The model under review builds one solid part; all positions refer to its coordinate system, in mm. Round coordinates to 2 decimals unless told otherwise and drop trailing zeros. Loops run counter-clockwise (first coordinate to the right, second up) from the corner with the lowest first, then second, coordinate; pieces in that order, holes last. Notation, with made-up numbers: (-28.75, -28.75) -> (-3.75, -28.75) arc R35 ccw to (-3.75, 4.25) -> close; hole circle Ø11 at (8, 79). An arc over 180 degrees is marked (long way). Write each question's results on one line, items separated by ' | '. Start each with the question number.
Item 1: Clearance check with a flat-ended pin moving along its axis: pin 1 Ø2.5 at (x, z) = (-3.5, -30.75) entering from -Y. State where the tip first meets the part, or that it passes through.
Item 2: For L1, parallel to X at y = 1.8, z = -55; L2, parallel to X at y = 1.3, z = -39.5; L3, parallel to Z at x = -3.25, y = 1.35, list the stretches that pass through material, from the lowest coordinate up. Write a range as from..to.
Item 3: We need section B-B (y = 1.95). Give the number of separate pieces and of enclosed holes in the cut face, and give its area (3 significant figures).
Item 4: We need section C-C (z = 27). Give the boundary of the cut face in (x, y) (3 decimals).
Item 5: We need section A-A (z = 39.5). Give the boundary of the cut face in (x, y) (3 decimals), and give its area (3 significant figures).
from build123d import *

# Parameters (mm, degrees)
BOSS_EXTRUDE1_DEPTH = 3.175
SKETCH2_W           = 3.175
SKETCH2_H           = 15
CUT_EXTRUDE1_DEPTH  = 62.928027782
SKETCH5_R           = 1.5
CUT_EXTRUDE2_DEPTH  = 10
FILLET1_R           = 2
FILLET2_R           = 3


with BuildPart() as part:
    # Sketch1 → Boss-Extrude1 (new body)
    with BuildSketch(Plane(origin=(0, 0, 0), x_dir=(1, 0, 0), z_dir=(0, 1, 0))):
        Polygon((-15, 60), (15, 60), (15, 45), (7, 45), (7, -45), (15, -45), (15, -60), (-15, -60), (-15, -45), (-7, -45), (-7, 45), (-15, 45), align=None)
    extrude(amount=BOSS_EXTRUDE1_DEPTH)

    # Sketch2 → Cut-Extrude1 (cut, through all)
    with BuildSketch(Plane(origin=(0, 3.175, 0), x_dir=(1, 0, 0), z_dir=(0, 1, 0))):
        with Locations((7.5, 60)):
            Rectangle(SKETCH2_W, SKETCH2_H)
        with Locations((-7.5, 60)):
            Rectangle(SKETCH2_W, SKETCH2_H)
        with Locations((7.5, -60)):
            Rectangle(SKETCH2_W, SKETCH2_H)
        with Locations((-7.5, -60)):
            Rectangle(SKETCH2_W, SKETCH2_H)
    extrude(amount=-CUT_EXTRUDE1_DEPTH, mode=Mode.SUBTRACT)

    # Sketch5 → Cut-Extrude2 (cut)
    with BuildSketch(Plane.XZ):
        with Locations(Location((3.5, -39.5, 0), (0, 0, 270))):
            Circle(SKETCH5_R)
        with Locations(Location((-3.5, -39.5, 0), (0, 0, 270))):
            Circle(SKETCH5_R)
        with Locations(Location((-3.5, -30.75, 0), (0, 0, 270))):
            Circle(SKETCH5_R)
        with Locations(Location((3.5, 30.75, 0), (0, 0, 270))):
            Circle(SKETCH5_R)
        with Locations(Location((-3.5, 30.75, 0), (0, 0, 270))):
            Circle(SKETCH5_R)
        with Locations(Location((3.5, 39.5, 0), (0, 0, 270))):
            Circle(SKETCH5_R)
        with Locations(Location((-3.5, 39.5, 0), (0, 0, 270))):
            Circle(SKETCH5_R)
        with Locations(Location((3.5, -30.75, 0), (0, 0, 270))):
            Circle(SKETCH5_R)
    extrude(amount=-CUT_EXTRUDE2_DEPTH, mode=Mode.SUBTRACT)

    # Fillet1
    fillet1_edges = [part.edges().sort_by_distance(p)[0] for p in [
        (-5.9125, 1.5875, -60),
        (-9.0875, 1.5875, -60),
        (5.9125, 1.5875, 60),
        (9.0875, 1.5875, 60),
        (-5.9125, 1.5875, 60),
        (-9.0875, 1.5875, 60),
        (9.0875, 1.5875, -60),
        (5.9125, 1.5875, -60),
    ]]
    fillet(fillet1_edges, radius=FILLET1_R)

    # Fillet2
    fillet2_edges = [part.edges().sort_by_distance(p)[0] for p in [
        (7, 1.5875, -45),
        (7, 1.5875, 45),
        (15, 1.5875, 45),
        (15, 1.5875, 60),
        (-15, 1.5875, 60),
        (-15, 1.5875, 45),
        (-7, 1.5875, 45),
        (-7, 1.5875, -45),
        (-15, 1.5875, -45),
        (-15, 1.5875, -60),
        (15, 1.5875, -60),
        (15, 1.5875, -45),
    ]]
    fillet(fillet2_edges, radius=FILLET2_R)


solid = part.part
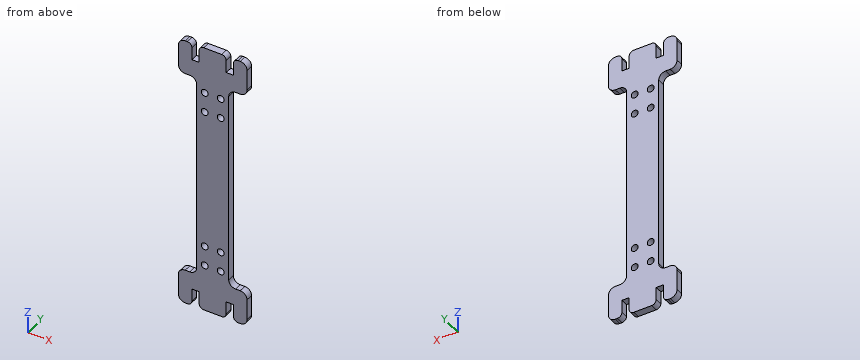
Here are the results:
1) pin 1: passes through
2) L1: x = -15..-9.09, -5.91..5.91, 9.09..15 | L2: x = -7..-5, -2..2, 5..7 | L3: z = -60..-40.98, -38.02..-32.23, -29.27..29.27, 32.23..38.02, 40.98..60
3) separate pieces: 1 | enclosed holes: 8 | area: 1,990 mm2
4) outline: (-7, 0) -> (7, 0) -> (7, 3.175) -> (-7, 3.175) -> close
5) outline: (-7, 0) -> (-5, 0) -> (-5, 3.175) -> (-7, 3.175) -> close; (-2, 0) -> (2, 0) -> (2, 3.175) -> (-2, 3.175) -> close; (5, 0) -> (7, 0) -> (7, 3.175) -> (5, 3.175) -> close | area: 25.4 mm2
